```python
from build123d import *

# Parameters (mm, degrees)
SKETCH1_W           = 36.322
SKETCH1_H           = 16.256
BOSS_EXTRUDE1_DEPTH = 2.032
SKETCH2_R           = 2.54
BOSS_EXTRUDE2_DEPTH = 17.78
FILLET1_R           = 2.54
FILLET2_R           = 2.54
FILLET3_R           = 1.27
SKETCH3_R           = 3.556
BOSS_EXTRUDE3_DEPTH = 5.08


with BuildPart() as part:
    # Sketch1 → Boss-Extrude1 (new body)
    with BuildSketch(Plane(origin=(0, 0, 0), x_dir=(1, 0, 0), z_dir=(0, 1, 0))):
        with Locations((18.161, -8.128)):
            Rectangle(SKETCH1_W, SKETCH1_H)
    extrude(amount=BOSS_EXTRUDE1_DEPTH)

    # Sketch2 → Boss-Extrude2 (add)
    with BuildSketch(Plane(origin=(0, 2.032, 0), x_dir=(1, 0, 0), z_dir=(0, 1, 0))):
        with Locations(Location((18.161, -8.128, 0), (0, 0, 270))):
            Circle(SKETCH2_R)
    extrude(amount=BOSS_EXTRUDE2_DEPTH)

    # Fillet1
    fillet1_edges = [part.edges().sort_by_distance(p)[0] for p in [
        (18.161, 19.812, 5.588),
    ]]
    fillet(fillet1_edges, radius=FILLET1_R)

    # Fillet2
    fillet2_edges = [part.edges().sort_by_distance(p)[0] for p in [
        (18.161, 2.032, 5.588),
    ]]
    fillet(fillet2_edges, radius=FILLET2_R)

    # Fillet3
    fillet3_edges = [part.edges().sort_by_distance(p)[0] for p in [
        (0, 1.016, 0),
        (36.322, 1.016, 0),
        (36.322, 1.016, 16.256),
        (0, 1.016, 16.256),
    ]]
    fillet(fillet3_edges, radius=FILLET3_R)

    # Sketch3 → Boss-Extrude3 (add)
    with BuildSketch(Plane.XZ):
        with Locations(Location((10.16, 8.128, 0), (0, 0, 90))):
            Circle(SKETCH3_R)
        with Locations(Location((26.162, 8.128, 0), (0, 0, 90))):
            Circle(SKETCH3_R)
    extrude(amount=BOSS_EXTRUDE3_DEPTH)


solid = part.part
```
Check sheet for the modelled part. Datum: model origin and axes. Units: mm. A direction names the side the tool comes from. Give positions to 0.01 mm unless a question says otherwise; leave off trailing zeros. Write each loop counter-clockwise with the first axis right and the second up, starting at its lowest first coordinate (ties: lowest second). Pieces come first, ordered by that corner, then holes.
Item 1: Cross-section at C-C (z = 14). Enter the section's corners in (x, y).
Item 2: Cross-section at B-B (y = -2.5). Enter the section's corners in (x, z), and give its area (3 significant figures).
Item 3: Gauge pin test, flat ends, axial feed: pin 1 (8 mm diameter, centred on y = 8.5, z = 14, fed in from -X); pin 2 (3 mm diameter, centred on y = 6, z = 9, fed in from +X); pin 3 (1 mm diameter, centred on y = 3, z = 7, fed in from +X). Record the tip position at first contact, or that the pin passes through.
Item 4: Scan lines: L1, parallel to Y at x = 9, z = 3.5; L2, parallel to Y at x = 25, z = 8.5; L3, parallel to Z at x = 10, y = -2.75. Record each from-to range of solid material in increasing order.
Item 5: Access from +Z, -Z, +X, -X, +Y, -Y to the whole of each face (thin tool, end or side, straight path). Record for faces 4 (the face through (18, 1, 0)), 5 (the face through (22.636, -2.504, 7.665)), 6 (the face through (20.3, 10.8, 9.5)).
Item 6: Cross-section at D-D (y = 18). Enter the section's corners in (x, z), and give its area (3 significant figures).
Item 7: Cross-section at A-A (x = 10.16). Enter the section's corners in (y, z).
Item 8: Draft check along X on faces 1 (the face through (7.16, -2.5, 10.04)), 2 (the face through (26, -5.08, 8)), 3 (the face through (35.94, 1.03, 0.36)). Enter one of: released by +X, released by -X, zero draft, split by the parting line, or undercut.
Report:
1. outline: (0, 0) - (36.32, 0) - (36.32, 2.03) - (0, 2.03) - close
2. outline: circle Ø7.11 at (10.16, 8.13); circle Ø7.11 at (26.16, 8.13)
2. area: 79.5 mm2
3. pin 1: stops at x = 16.44
3. pin 2: stops at x = 20.7
3. pin 3: stops at x = 21.61
4. L1: y = 0 to 2.03
4. L2: y = -5.08 to 2.03
4. L3: z = 4.58 to 11.68
5. face 4: -Z, +X, -X, +Y, -Y
5. face 5: -Y
5. face 6: +Y
6. outline: circle Ø4.87 at (18.16, 8.13)
6. area: 18.6 mm2
7. outline: (-5.08, 4.57) - (0, 4.57) - (0, 0) - (2.03, 0) - (2.03, 16.26) - (0, 16.26) - (0, 11.68) - (-5.08, 11.68) - close
8. face 1: undercut
8. face 2: zero draft
8. face 3: released by +X
